Autodesk Inventor part; units mm, degrees
ref_plane "YZ Plane" through (0, 0, 0) normal (1, 0, 0) x (0, 1, 0)
ref_plane "XZ Plane" through (0, 0, 0) normal (0, 1, 0) x (-1, 0, 0)
ref_plane "XY Plane" through (0, 0, 0) normal (0, 0, 1) x (1, 0, 0)
sketch "Sketch1" plane through (0, 0, 0) normal (0, 0, 1) x (1, 0, 0)
  line L0 (-50, -55) -> (50, -55)
  line L1 (50, -55) -> (50, 55)
  line L2 (50, 55) -> (-50, 55)
  line L3 (-50, 55) -> (-50, -55)
  line L4 (-50, -55) -> (50, 55) construction
  line L5 (50, -55) -> (-50, 55) construction
  point P0 (0, 0)
  dimension "d0" = 100
  dimension "d1" = 110
extrude "Plate1" add sketch "Sketch1" along normal blind 6
fillet "Corner Round1" radius 20 4 edges at (50, -55, 3) (-50, -55, 3) (-50, 55, 3) (50, 55, 3)
sketch "Sketch5" plane through (0, 0, 6) normal (0, 0, 1) x (1, 0, 0)
  line L0 (50, 35) -> (50, -35)
  line L1 (50, 25) -> (-50, 25)
  line L2 (-50, -35) -> (-50, 35)
  line L3 (-30, 55) -> (30, 55)
  point P0 (0, 0)
  dimension "d23" = 30
feature "Fold1" [suppressed]
equation "\"d2\" = Thickness"
equation "\"d24\" = BendReliefWidth"
equation "\"d25\" = BendReliefDepth"
equation "\"d26\" = MinimumRemnant"
equation "\"d27\" = TransitionRadius"
equation "\"d29\" = BendRadius"
equation "\"BendReliefWidth\" = Thickness"
equation "\"BendReliefDepth\" = 0.5 * Thickness"
equation "\"CornerReliefSize\" = 4 * Thickness"
equation "\"MinimumRemnant\" = 2 * Thickness"
equation "\"TransitionRadius\" = BendRadius"
equation "\"JacobiRadiusSize\" = BendRadius"
equation "\"GapSize\" = Thickness"
properties part number "PRS 940-93 leg plate for filter" material "Stainless Steel"
Geometry: final body of the model. Coordinates: model frame, mm. Give positions to 0.01 mm unless a question says otherwise; leave off trailing zeros. Order: outer loops, then holes, each group sorted by start corner. A loop starts at its lowest first (then second) coordinate and runs counter-clockwise, first axis right, second up. Notation, with made-up numbers: (76, -35) -> (100, -35) arc R29 cw to (100, 1) -> close; hole circle Ø2 at (34.5, 36). An arc over 180 degrees is marked (long way). Answer as a JSON object with one key per item and string values.
Q1. Section A-A (z = 2.2). Output: boundary loops of the cut face in (x, y).
Entries:
{"outline": "(-50, -35) arc R20 ccw to (-30, -55) -> (30, -55) arc R20 ccw to (50, -35) -> (50, 35) arc R20 ccw to (30, 55) -> (-30, 55) arc R20 ccw to (-50, 35) -> close"}
Q2. Section C-C (y = -44). Output: boundary loops of the cut face in (x, z), plus the area to 3 significant figures.
Entries:
{"outline": "(-47.86, 0) -> (47.86, 0) -> (47.86, 6) -> (-47.86, 6) -> close", "area": "574 mm^2"}
Q3. First-contact query: pin 1 (5 mm diameter, centred on x = 38, y = -41, fed in from -Z). Flat tip, straight axial feed; report the tip coordinate or a pass-through.
Entries:
{"pin 1": "stops at z = 0"}
Q4. Section B-B (x = 43). Output: boundary loops of the cut face in (y, z).
Entries:
{"outline": "(-50.2, 0) -> (50.2, 0) -> (50.2, 6) -> (-50.2, 6) -> close"}
Q5. Material intervals for probe 1 along X at (y, z) = (-48.5, 4.1); probe 2 along X at (y, z) = (49.5, 2.8); probe 3 along Y at (x, z) = (-40, 3.95), sorted ascending.
Entries:
{"probe 1": "x = -44.76 to 44.76", "probe 2": "x = -43.77 to 43.77", "probe 3": "y = -52.32 to 52.32"}
